Design review of the part built by this model. Coordinates are the model's own, in mm. A direction names the side the tool comes from. Coordinates: 2 decimals unless noted, no trailing zeros. Write each loop counter-clockwise with the first axis right and the second up, starting at its lowest first coordinate (ties: lowest second). Pieces come first, ordered by that corner, then holes. Notation, with made-up numbers: (33.25, -24.5) - (83.25, -24.5) arc R30 cw to (83.25, 13.5) - close; hole circle Ø7 at (-14.75, 74.25). An arc over 180 degrees is marked (long way). Answer as a JSON object with one key per item and string values.
```python
from build123d import *

# Parameters (mm, degrees)
BOSS_EXTRUDE1_DEPTH          = 3.175
FILLET1_R                    = 6.35
F_10_0_1935_DIAMETER_HOLE1_D = 4.9149


with BuildPart() as part:
    # Sketch1 → Boss-Extrude1 (new body)
    with BuildSketch(Plane.XY):
        Polygon((0, 0), (0, 50.8), (-25.4, 50.8), (-25.4, 38.870384182), (-38.870384182, 25.4), (-76.2, 25.4), (-76.2, 0), align=None)
    extrude(amount=BOSS_EXTRUDE1_DEPTH)

    # Fillet1
    fillet1_edges = [part.edges().sort_by_distance(p)[0] for p in [
        (-76.2, 0, 1.5875),
        (-76.2, 25.4, 1.5875),
        (-38.870384182, 25.4, 1.5875),
        (-25.4, 38.870384182, 1.5875),
        (-25.4, 50.8, 1.5875),
        (0, 50.8, 1.5875),
        (0, 0, 1.5875),
    ]]
    fillet(fillet1_edges, radius=FILLET1_R)

    # #10 (0.1935) Diameter Hole1 (through all)
    with Locations(Plane.XY.offset(3.175)):
        with Locations((-63.5, 12.7), (-50.8, 12.7), (-12.7, 25.4), (-12.7, 38.1), (-38.1, 12.7), (-12.7, 12.7)):
            Hole(F_10_0_1935_DIAMETER_HOLE1_D / 2)


solid = part.part
```
(1) Take a section at C-C, the plane x = -12.7. Write out the cut boundary in (y, z) (3 decimals).
Solved:
{"outline": "(0, 0) - (10.243, 0) - (10.243, 3.175) - (0, 3.175) - close; (15.157, 0) - (22.943, 0) - (22.943, 3.175) - (15.157, 3.175) - close; (27.857, 0) - (35.643, 0) - (35.643, 3.175) - (27.857, 3.175) - close; (40.557, 0) - (50.8, 0) - (50.8, 3.175) - (40.557, 3.175) - close"}
(2) For pin 1 (4.5 mm diameter, centred on x = -12.7, y = 25.4, fed in from -Z); pin 2 (1.6 mm diameter, centred on x = -58, z = 1, fed in from +Y); pin 3 (0.9 mm diameter, centred on y = 43.5, z = 2, fed in from -X), all flat-tipped, find the tip position at first contact; note any pin that passes through.
Solved:
{"pin 1": "passes through", "pin 2": "stops at y = 25.4", "pin 3": "stops at x = -25.4"}
(3) Take a section at A-A, the plane x = -50.8. Write out the cut boundary in (y, z) (3 decimals), and give its area (3 significant figures).
Solved:
{"outline": "(0, 0) - (10.243, 0) - (10.243, 3.175) - (0, 3.175) - close; (15.157, 0) - (25.4, 0) - (25.4, 3.175) - (15.157, 3.175) - close", "area": "65.0 mm^2"}
(4) Take a section at D-D, the plane y = 39. Write out the cut boundary in (x, z) (3 decimals).
Solved:
{"outline": "(-25.913, 0) - (-14.987, 0) - (-14.987, 3.175) - (-25.913, 3.175) - close; (-10.413, 0) - (0, 0) - (0, 3.175) - (-10.413, 3.175) - close"}
(5) Take a section at B-B, the plane z = 1.9. Write out the cut boundary in (x, y).
Solved:
{"outline": "(-76.2, 6.35) arc R6.35 ccw to (-69.85, 0) - (-6.35, 0) arc R6.35 ccw to (0, 6.35) - (0, 44.45) arc R6.35 ccw to (-6.35, 50.8) - (-19.05, 50.8) arc R6.35 ccw to (-25.4, 44.45) - (-25.4, 41.5) arc R6.35 cw to (-27.26, 37.01) - (-37.01, 27.26) arc R6.35 cw to (-41.5, 25.4) - (-69.85, 25.4) arc R6.35 ccw to (-76.2, 19.05) - close; hole circle Ø4.91 at (-63.5, 12.7); hole circle Ø4.91 at (-50.8, 12.7); hole circle Ø4.91 at (-38.1, 12.7); hole circle Ø4.91 at (-12.7, 12.7); hole circle Ø4.91 at (-12.7, 25.4); hole circle Ø4.91 at (-12.7, 38.1)"}
(6) To check wall thickness, follow line 1 (Y direction, x = -12.7, z = 0.7); line 2 (Y direction, x = -13, z = 0.6); line 3 (Y direction, x = -51, z = 2.9). State the ranges of each line that lie inside material, in increasing order. Write a range as from..to.
Solved:
{"line 1": "y = 0..10.24, 15.16..22.94, 27.86..35.64, 40.56..50.8", "line 2": "y = 0..10.26, 15.14..22.96, 27.84..35.66, 40.54..50.8", "line 3": "y = 0..10.25, 15.15..25.4"}
(7) Tool access review of faces 1 (the face through (-36.29, 14.36, 1.57)), 2 (the face through (-25.4, 43, 2)): name each direction out of +Z, -Z, +X, -X, +Y, -Y from which nothing blocks a thin tool from reaching the whole face with its end or side.
Solved:
{"face 1": "+Z, -Z", "face 2": "+Z, -Z, -X, +Y"}
(8) The part is to be moulded in two halves that separate along X. For faces 3 (the face through (-15.044, 13.438, 1.565)), 4 (the face through (0, 25, 2)), 5 (the face through (-14.97, 24.46, 1.57)), 6 (the face through (-32.07, 32.2, 1.57)), say which applies: pulls with the +X half, pulls with the -X half, needs draft (parallel to the pull), parting line crosses it, or undercut.
Solved:
{"face 3": "undercut", "face 4": "pulls with the +X half", "face 5": "undercut", "face 6": "pulls with the -X half"}
